```python
from build123d import *

# Parameters (mm, degrees)
SKETCH1_W                      = 23
SKETCH1_H                      = 10
HOLE1_D                        = 40
HOLE1_DEPTH                    = 5.8
SKETCH4_W                      = 12.5
SKETCH4_H                      = 5.8
M4X0_7_TAPPED_HOLE1_D          = 3.3
CBORE_FOR_M6_SHCS1_D           = 7
CBORE_FOR_M6_SHCS1_CBORE_D     = 11
CBORE_FOR_M6_SHCS1_CBORE_DEPTH = 6.5
FILLET1_R                      = 4


with BuildPart() as part:
    # Sketch1 → Revolve1 (revolve)
    with BuildSketch(Plane.XZ, mode=Mode.PRIVATE) as revolve1_sk:
        with Locations((11.5, 5)):
            Rectangle(SKETCH1_W, SKETCH1_H)
    revolve(revolve1_sk.sketch.rotate(Axis((0, 0, 10), (0, 0, -1)), 180), axis=Axis((0, 0, 10), (0, 0, -1)))

    # Hole1
    with Locations(Plane(origin=(0, 0, 0), x_dir=(-1, 0, 0), z_dir=(0, 0, -1))):
        with Locations((0, 0)):
            Hole(HOLE1_D / 2, depth=HOLE1_DEPTH)

    # Sketch4 → Revolve2 (revolve)
    with BuildSketch(Plane.XZ, mode=Mode.PRIVATE) as revolve2_sk:
        with Locations((6.25, 2.9)):
            Rectangle(SKETCH4_W, SKETCH4_H)
    revolve(revolve2_sk.sketch.rotate(Axis((0, 0, 5.8), (0, 0, -1)), 180), axis=Axis((0, 0, 5.8), (0, 0, -1)))

    # M4x0.7 Tapped Hole1 (through all)
    with Locations(Plane(origin=(0, 0, 5.8), x_dir=(-1, 0, 0), z_dir=(0, 0, -1))):
        with Locations((-14.072912811, 8.125), (-14.072912811, -8.125), (0, -16.25), (14.072912811, -8.125), (14.072912811, 8.125), (0, 16.25)):
            Hole(M4X0_7_TAPPED_HOLE1_D / 2)

    # CBORE for M6 SHCS1 (through all)
    with Locations(Plane.XY.offset(10)):
        with Locations((0, 0)):
            CounterBoreHole(CBORE_FOR_M6_SHCS1_D / 2, CBORE_FOR_M6_SHCS1_CBORE_D / 2, CBORE_FOR_M6_SHCS1_CBORE_DEPTH)

    # Fillet1
    fillet1_edges = [part.edges().sort_by_distance(p)[0] for p in [
        (23, 0, 10),
    ]]
    fillet(fillet1_edges, radius=FILLET1_R)


solid = part.part
```
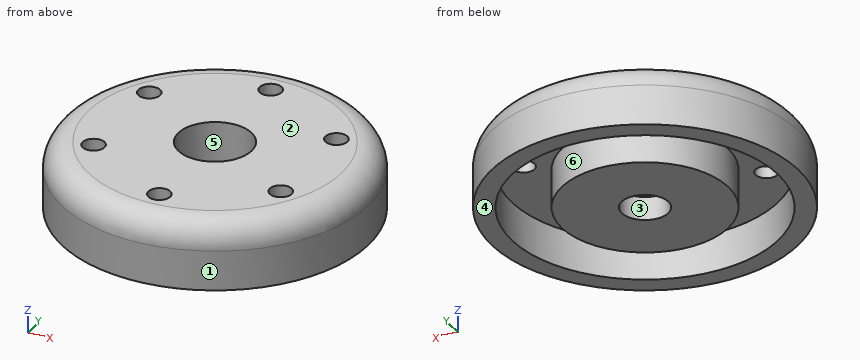
Verification items for the finished model (mm, model axes). Face numbers are marked on the shaded views. A direction names the side the tool comes from. Give positions to 0.01 mm unless a question says otherwise; leave off trailing zeros. Write each loop counter-clockwise with the first axis right and the second up, starting at its lowest first coordinate (ties: lowest second). Pieces come first, ordered by that corner, then holes. Notation, with made-up numbers: M 72,-13 L 109,-13 A15 ccw 109,-3 Z; hole C 46,59.5 d6. An arc over 180 degrees is marked long. One line per question, with ' | ' between items.
1) Section check B-B on x = 0. State how many separate pieces and enclosed holes the cut face has, plus the area to 3 significant figures.
Result:
separate pieces: 4 | enclosed holes: 0 | area: 242 mm2
2) Set-up check for the marked faces 4, 5 and 6: record each of +Z, -Z, +X, -X, +Y, -Y from which the full face is reachable in a straight line by a thin tool's end or side.
Result:
face 4: -Z, +X, -X, +Y, -Y | face 5: +Z | face 6: -Z
3) Section check C-C on z = 2.25. Enter the section's corners in (x, y).
Result:
outline: C 0,0 d46; C 0,0 d25; hole C 0,0 d40; hole C 0,0 d7
4) Gauge pin test, flat ends, axial feed: pin 1 Ø6 at (y, z) = (-15, 1) entering from +X; pin 2 Ø4 at (x, y) = (-9, -8) entering from -Z; pin 3 Ø4 at (x, y) = (-3.5, -17) entering from -Z; pin 4 Ø2 at (x, y) = (0, -16.25) entering from +Z. Record the tip position at first contact, or that the pin passes through.
Result:
pin 1: stops at x = 19.62 | pin 2: stops at z = 0 | pin 3: stops at z = 5.8 | pin 4: passes through
5) Thickness scan on line 1 along Y through (x, z) = (0, 1.1); line 2 along X through (y, z) = (1.5, 1.5). Record the ranges inside material, lowest first. Write a range as [from, to].
Result:
line 1: y = [-23, -20], [-12.5, -3.5], [3.5, 12.5], [20, 23] | line 2: x = [-22.95, -19.94], [-12.41, -3.16], [3.16, 12.41], [19.94, 22.95]
6) Section check A-A on y = 0. Enter the section's corners in (x, z).
Result:
outline: M -23,0 L -20,0 L -20,5.8 L -12.5,5.8 L -12.5,0 L -3.5,0 L -3.5,3.5 L -5.5,3.5 L -5.5,10 L -19,10 A4 ccw -23,6 Z; M 3.5,0 L 12.5,0 L 12.5,5.8 L 20,5.8 L 20,0 L 23,0 L 23,6 A4 ccw 19,10 L 5.5,10 L 5.5,3.5 L 3.5,3.5 Z
7) Mould release check, pull along X, two halves, no side actions. Record for the marked faces 1, 2 and 3: released by +X, released by -X, zero draft, split by the parting line, or undercut.
Result:
face 1: split by the parting line | face 2: zero draft | face 3: undercut
8) Section check D-D on z = 5.25. Enter the section's corners in (x, y).
Result:
outline: C 0,0 d46; C 0,0 d25; hole C 0,0 d40; hole C 0,0 d11
